Autodesk Inventor part; units mm, degrees
ref_plane "YZ Plane" through (0, 0, 0) normal (1, 0, 0) x (0, 1, 0)
ref_plane "XY Plane" through (0, 0, 0) normal (0, 0, 1) x (1, 0, 0)
sketch "Sketch1" plane through (0, 0, 0) normal (0, 0, 1) x (1, 0, 0)
  line L0 (0, 0) -> (609.6, 0)
  line L1 (609.6, 0) -> (609.6, 317.881)
  line L2 (609.6, 317.881) -> (0, 317.881)
  line L3 (0, 317.881) -> (0, 0)
  dimension "d0" = 609.6
  dimension "d1" = 317.881
extrude "Extrusion1" add sketch "Sketch1" along normal blind 5.7658
sketch "Sketch2" plane through (0, 317.881, 0) normal (0, 1, 0) x (1, 0, 0)
  line L0 (609.6, 0) -> (0, 0)
  line L1 (0, 0) -> (0, -5.7658)
  line L2 (609.6, -5.7658) -> (0, -5.7658)
  line L3 (609.6, 0) -> (609.6, -5.7658)
  line L4 (0, 0) -> (609.6, 0)
  line L5 (0, 0) -> (14.4594, -5.7658)
  line L6 (0, -5.7658) -> (609.6, -5.7658)
  line L7 (14.4594, -5.7658) -> (14.4594, 0)
  line L8 (14.4594, -5.7658) -> (20.2252, -5.7658) construction
  dimension "d4" = 21.74
  dimension "d5" = 90
extrude "Extrusion2" cut sketch "Sketch2" against normal through all contours L5 L2 L1
sketch "Sketch3" plane through (609.6, 0, 0) normal (1, 0, 0) x (0, 0, -1)
  line L0 (0, 0) -> (0, 317.881)
  line L1 (0, 317.881) -> (-5.7658, 317.881)
  line L2 (-5.7658, 0) -> (-5.7658, 317.881)
  line L3 (0, 0) -> (-5.7658, 0)
  line L4 (0, 0) -> (-5.7658, 0)
  line L5 (0, 0) -> (-5.7658, 5.7658)
  line L6 (-5.7658, 0) -> (-5.7658, 317.881)
  line L7 (0, 0) -> (8.1541, 0) construction
  line L8 (0, 317.881) -> (-5.7658, 317.881)
  line L9 (0, 317.881) -> (-5.7658, 312.1152)
  line L10 (0, 317.881) -> (8.1541, 317.881) construction
  dimension "d8" = 135
  dimension "d9" = 135
extrude "Extrusion3" cut sketch "Sketch3" against normal through all contours L3 L2 L5 | L9 L2 L1
ref_plane "Work Plane1" through (0, 158.9405, 0) normal (0, 1, 0) x (-1, 0, 0)
sketch "Sketch4" plane through (0, 158.9405, 0) normal (0, 1, 0) x (-1, 0, 0)
  line L0 (-14.4594, 5.7658) -> (0, 0)
  line L1 (-609.6, 5.7658) -> (-14.4594, 5.7658)
  line L2 (-609.6, 0) -> (-609.6, 5.7658)
  line L3 (-609.6, 0) -> (0, 0)
  line L4 (-609.6, 5.7658) -> (-584.2, 5.7658) construction
  line L5 (-584.2, 5.7658) -> (-609.6, 4.4413)
  point P0 (0, 0)
  dimension "d13" = 25.4
  dimension "d14" = 2.985
extrude "Extrusion4" cut sketch "Sketch4" against normal through all both and the other way through all contours L5 L2 L1
properties part number "Wind Tunnel Test Section Back" material "Polycarbonate, Clear"
Geometry check sheet. Reference: the model listing, model coordinates, mm. Round coordinates to 2 decimals unless told otherwise and drop trailing zeros. Order: outer loops, then holes, each group sorted by start corner. A loop starts at its lowest first (then second) coordinate and runs counter-clockwise, first axis right, second up. Notation, with made-up numbers: (86.25, 17.5) - (144.25, 17.5) arc R11 ccw to (144.25, 25.5) - close; hole circle Ø3 at (-29, 18). An arc over 180 degrees is marked (long way). Use a Markdown table: item, result. Add a question column.
(1) Sectioned sample at C-C, the plane z = 2.35. Enter the section's corners in (x, y).
(2) Sectioned sample at B-B, the plane x = 216. Enter the section's corners in (y, z), and give its area (3 significant figures).
(3) Material ranges on line 1 along Y through (x, z) = (392, 2.4); line 2 along Y through (x, z) = (359, 0.25), recorded low to high. Write a range as [from, to].
(4) Depth check by flat-ended pin: pin 1 (1.5 mm diameter, centred on x = 157.5, z = 3.5, fed in from +Y). Enter the tip coordinate at first touch or a pass-through.
(5) Sectioned sample at A-A, the plane y = 116.5. Enter the section's corners in (x, z), and give its area (3 significant figures).
Answers below:
| question | item | result |
|---|---|---|
| 1 | outline | (5.89, 2.35) - (609.6, 2.35) - (609.6, 315.53) - (5.89, 315.53) - close |
| 2 | outline | (0, 0) - (317.88, 0) - (312.12, 5.77) - (5.77, 5.77) - close |
| 2 | area | 1,800 mm² |
| 3 | line 1 | [2.4, 315.48] |
| 3 | line 2 | [0.25, 317.63] |
| 4 | pin 1 | y = 315.13 |
| 5 | outline | (0, 0) - (609.6, 0) - (609.6, 4.44) - (584.2, 5.77) - (14.46, 5.77) - close |
| 5 | area | 3,460 mm² |
